from build123d import *

# Parameters (mm, degrees)
SKETCH_1_R               = 30
EXTRUDE_1_DEPTH          = 4
SKETCH_2_R               = 2.1
CUT_EXTRUDE_1_DEPTH      = 4
PATTERN_CIRCULAR_1_COUNT = 3
SKETCH_3_R               = 6.6
CUT_EXTRUDE_2_DEPTH      = 17
SKETCH_4_R               = 1.6
CUT_EXTRUDE_3_DEPTH      = 17
PATTERN_CIRCULAR_2_COUNT = 3


with BuildPart() as part:
    # 草图1 → 凸台-拉伸1 (new body)
    with BuildSketch(Plane(origin=(0, 0, 0), x_dir=(1, 0, 0), z_dir=(0, 1, 0))):
        with Locations(Location((0, 0, 0), (0, 0, 270))):
            Circle(SKETCH_1_R)
    extrude(amount=EXTRUDE_1_DEPTH)

    # 草图2 → 切除-拉伸1 (cut)
    with BuildSketch(Plane(origin=(0, 4, 0), x_dir=(1, 0, 0), z_dir=(0, 1, 0))):
        with Locations(Location((0, 25, 0), (0, 0, 270))):
            Circle(SKETCH_2_R)
    cut_extrude_1 = extrude(amount=-CUT_EXTRUDE_1_DEPTH, mode=Mode.SUBTRACT)

    # 阵列(圆周)1: 切除-拉伸1 ×3 about axis
    pattern_circular_1_axis = Axis((0, 0, 0), (0, 1, 0))
    for i in range(1, PATTERN_CIRCULAR_1_COUNT):
        add(cut_extrude_1.rotate(pattern_circular_1_axis, i * 360 / PATTERN_CIRCULAR_1_COUNT), mode=Mode.SUBTRACT)

    # 草图3 → 切除-拉伸2 (cut)
    with BuildSketch(Plane(origin=(0, 4, 0), x_dir=(1, 0, 0), z_dir=(0, 1, 0))):
        with Locations(Location((0, 0, 0), (0, 0, 270))):
            Circle(SKETCH_3_R)
    extrude(amount=-CUT_EXTRUDE_2_DEPTH, mode=Mode.SUBTRACT)

    # 草图4 → 切除-拉伸3 (cut)
    with BuildSketch(Plane(origin=(0, 4, 0), x_dir=(1, 0, 0), z_dir=(0, 1, 0))):
        with Locations(Location((8.227241336, -4.75, 0), (0, 0, 270))):
            Circle(SKETCH_4_R)
    cut_extrude_3 = extrude(amount=-CUT_EXTRUDE_3_DEPTH, mode=Mode.SUBTRACT)

    # 阵列(圆周)2: 切除-拉伸3 ×3 about axis
    pattern_circular_2_axis = Axis((0, 0, 0), (0, 1, 0))
    for i in range(1, PATTERN_CIRCULAR_2_COUNT):
        add(cut_extrude_3.rotate(pattern_circular_2_axis, i * 360 / PATTERN_CIRCULAR_2_COUNT), mode=Mode.SUBTRACT)


solid = part.part
Read the model definition and answer for the solid it produces. Units are mm, in the model's axes. Give positions to 0.01 mm unless a question says otherwise; leave off trailing zeros. Loops run counter-clockwise (first coordinate to the right, second up) from the corner with the lowest first, then second, coordinate; pieces in that order, holes last. Notation, with made-up numbers: (41, -30) -> (47, -30) arc R28 ccw to (47, 6) -> close; hole circle Ø4 at (63, 6.5). An arc over 180 degrees is marked (long way). Use a Markdown table: item, result.
Q1. Section C-C, the plane z = 12.5 is taken. Determine the outline of the cut face in (x, y), then the cut area to 3 significant figures.
Solved:
| item | result |
|---|---|
| outline | (-27.27, 0) -> (-23.75, 0) -> (-23.75, 4) -> (-27.27, 4) -> close; (-19.55, 0) -> (19.55, 0) -> (19.55, 4) -> (-19.55, 4) -> close; (23.75, 0) -> (27.27, 0) -> (27.27, 4) -> (23.75, 4) -> close |
| area | 185 mm^2 |
Q2. Section B-B, the plane x = 0 is taken. Determine the outline of the cut face in (y, z), then the cut area to 3 significant figures.
Solved:
| item | result |
|---|---|
| outline | (0, -30) -> (4, -30) -> (4, -27.1) -> (0, -27.1) -> close; (0, -22.9) -> (4, -22.9) -> (4, -11.1) -> (0, -11.1) -> close; (0, -7.9) -> (4, -7.9) -> (4, -6.6) -> (0, -6.6) -> close; (0, 6.6) -> (4, 6.6) -> (4, 30) -> (0, 30) -> close |
| area | 158 mm^2 |
Q3. Each of these flat-tipped pins is pushed along its axis until it touches: pin 1 (2.5 mm diameter, centred on x = -8.23, z = 4.75, fed in from +Y); pin 2 (1.5 mm diameter, centred on y = 3, z = 8, fed in from -X); pin 3 (5 mm diameter, centred on x = 8.23, z = 4.75, fed in from +Y). Where does it stop, or does it pass through?
Solved:
| item | result |
|---|---|
| pin 1 | passes through |
| pin 2 | stops at x = -29.11 |
| pin 3 | stops at y = 4 |
Q4. Determine the mould class of faces 1 (the face through (1.32, 1.97, -29.97)), 2 (the face through (0, 4, -7)), 3 (the face through (-4.016, 2.028, -5.238)) for opening direction X: pulls with the +X half, pulls with the -X half, needs draft (parallel to the pull), parting line crosses it, or undercut.
Solved:
| item | result |
|---|---|
| face 1 | parting line crosses it |
| face 2 | needs draft |
| face 3 | undercut |
Q5. Find the intervals of material crossed by line 1 along X through (y, z) = (3.2, 0); line 2 along X through (y, z) = (1.1, 4.75); line 3 along X through (y, z) = (1.75, -25), in increasing order.
Solved:
| item | result |
|---|---|
| line 1 | x = -30 to -6.6, 6.6 to 30 |
| line 2 | x = -29.62 to -9.83, -6.63 to -4.58, 4.58 to 6.63, 9.83 to 29.62 |
| line 3 | x = -16.58 to -2.1, 2.1 to 16.58 |
Q6. Section A-A, the plane z = 0 is taken. Determine the outline of the cut face in (x, y).
Solved:
| item | result |
|---|---|
| outline | (-30, 0) -> (-6.6, 0) -> (-6.6, 4) -> (-30, 4) -> close; (6.6, 0) -> (30, 0) -> (30, 4) -> (6.6, 4) -> close |
Q7. Section D-D, the plane x = 23 is taken. Determine the outline of the cut face in (y, z), then the cut area to 3 significant figures.
Solved:
| item | result |
|---|---|
| outline | (0, -19.26) -> (4, -19.26) -> (4, 10.89) -> (0, 10.89) -> close; (0, 14.11) -> (4, 14.11) -> (4, 19.26) -> (0, 19.26) -> close |
| area | 141 mm^2 |
